Part model, mm, in its own coordinate system. A direction names the side the tool comes from. Round coordinates to 2 decimals unless told otherwise and drop trailing zeros. Loops run counter-clockwise (first coordinate to the right, second up) from the corner with the lowest first, then second, coordinate; pieces in that order, holes last. Notation, with made-up numbers: M 52,76.5 L 100,76.5 A36 cw 100,112.5 Z; hole C 83,12 d10. An arc over 180 degrees is marked long. Put each result on its own line as item: value. Start each with the question number.
1) Slice it at A-A on y = -114.5. Give the cut face in (x, z).
2) Which spindle directions (+Z, -Z, +X, -X, +Y, -Y) get a long thin tool onto all of the face, cutting with end or side? Do faces 4 (the flat face through (-44.999, -174, 21)), 5 (the flat face through (-84.999, -174, 20)), 6 (the cylindrical face through (-133.47, -115.27, 21.75)), 7 (the flat face through (-85.999, 4, 21)), 8 (the flat face through (-10, -130.481, 3)). Say none if no direction does.
3) Pull direction Y, two halves, no side cores. Call faces 1 (the flat face through (-75, -104, 15)), 2 (the cylindrical face through (-110.353, -64.656, 3.372)), 3 (the cylindrical face through (-142.69, -115.27, 1.6)): +Y half, -Y half, draft (parallel to the pull), parting line (faces both ways), or undercut.
4) Slice it at D-D on y = -136.5. Give the cut face in (x, z), then the cut area to 3 significant figures.
5) Slice it at C-C on x = -158. Give the cut face in (y, z).
6) Probe line 1 along Y through (x, z) = (-78, 43.5); line 2 along Z through (x, y) = (-26, -109); line 3 along X through (y, z) = (-83.5, 37). List the from-to ranges inside material, lowest first.
7) Slice it at B-B on y = -67.5. Give the cut face in (x, z).
8) Drop flat-ended pins along their axis: pin 1 Ø5.5 at (y, z) = (-101, 5) entering from -X; pin 2 Ø3.5 at (x, z) = (-9.5, 4.5) entering from -Y; pin 3 Ø12 at (y, z) = (-172, 25) entering from +X. Give the stop position or say it passes through.
```python
from build123d import *

# Parameters (mm, degrees)
EXTRUDE_1_DEPTH     = 6.84
EXTRUDE_2_DEPTH     = 12
SKETCH_3_R          = 26.5
EXTRUDE_3_DEPTH     = 48.5
SKETCH_4_R          = 31.5
EXTRUDE_4_DEPTH     = 5.63
SKETCH_5_R          = 21
CUT_EXTRUDE_1_DEPTH = 9.13
SKETCH_6_R          = 21
CUT_EXTRUDE_2_DEPTH = 2.92
SKETCH_7_R          = 16
SKETCH_9_R          = 21
SKETCH_8_R          = 16
SKETCH_10_R         = 17
CUT_EXTRUDE_3_DEPTH = 13.29
SKETCH_11_R         = 6
CUT_EXTRUDE_4_DEPTH = 42.92
EXTRUDE_5_DEPTH     = 15
SKETCH_13_R         = 5.5
CUT_EXTRUDE_5_DEPTH = 15
EXTRUDE_6_DEPTH     = 15
SKETCH_16_R         = 5.5
CUT_EXTRUDE_6_DEPTH = 15


with BuildPart() as part:
    # 스케치1 → 보스-돌출1 (new body)
    with BuildSketch(Plane.XY):
        with BuildLine():
            Line((-34.998826986, -181.181097978), (-34.998826986, -140.481097978))
            ThreePointArc((-34.998826986, -140.481097978), (-32.069894798, -133.410030166), (-24.998826986, -130.481097978))
            Line((-24.998826986, -130.481097978), (5.001173014, -130.481097978))
            Line((5.001173014, -130.481097978), (5.001173014, -47.181097978))
            Line((5.001173014, -47.181097978), (-25.998826986, -47.181097978))
            ThreePointArc((-25.998826986, -47.181097978), (-33.069894798, -44.25216579), (-35.998826986, -37.181097978))
            Line((-35.998826986, -37.181097978), (-35.998826986, 11.818902022))
            Line((-35.998826986, 11.818902022), (-95.998826986, 11.818902022))
            Line((-95.998826986, 11.818902022), (-95.998826986, -48.181097978))
            ThreePointArc((-95.998826986, -48.181097978), (-110.502915378, -64.929776001), (-116.68226469, -86.206581157))
            Line((-116.68226469, -86.206581157), (-116.68226469, -87.311097978))
            Line((-116.68226469, -87.311097978), (-134.998826986, -87.311097978))
            Line((-134.998826986, -87.311097978), (-134.998826986, -121.181097978))
            Line((-134.998826986, -121.181097978), (-104.998826986, -121.181097978))
            ThreePointArc((-104.998826986, -121.181097978), (-97.927759174, -124.110030166), (-94.998826986, -131.181097978))
            Line((-94.998826986, -131.181097978), (-94.998826986, -181.181097978))
            Line((-94.998826986, -181.181097978), (-34.998826986, -181.181097978))
        make_face()
    extrude(amount=EXTRUDE_1_DEPTH)

    # 스케치2 → 보스-돌출2 (add)
    with BuildSketch(Plane.XZ.offset(121.181097978)):
        with BuildLine():
            Line((-114.998826986, 0), (-114.998826986, 15.74))
            ThreePointArc((-114.998826986, 15.74), (-116.46329308, 19.275533906), (-119.998826986, 20.74))
            Line((-119.998826986, 20.74), (-129.093412943, 20.74))
            ThreePointArc((-129.093412943, 20.74), (-133.528440233, 21.777269783), (-137.043403564, 24.673893413))
            Line((-137.043403564, 24.673893413), (-164.048836366, 60.066106587))
            ThreePointArc((-164.048836366, 60.066106587), (-178.064933574, 61.949990621), (-179.948817607, 47.933893413))
            Line((-179.948817607, 47.933893413), (-147.876203482, 5.900840119))
            ThreePointArc((-147.876203482, 5.900840119), (-142.603758486, 1.555904675), (-135.951217551, 0))
            Line((-135.951217551, 0), (-114.998826986, 0))
        make_face()
    extrude(amount=-EXTRUDE_2_DEPTH)

    # 스케치3 → 보스-돌출3 (add)
    with BuildSketch(Plane.XY.offset(6.84)):
        with Locations(Location((-64.998826986, -91.181097978, 0), (0, 0, 180))):
            Circle(SKETCH_3_R)
    extrude(amount=EXTRUDE_3_DEPTH)

    # 스케치4 → 보스-돌출4 (add)
    with BuildSketch(Plane.XY.offset(6.84)):
        with Locations((-64.998826986, -91.181097978)):
            Circle(SKETCH_4_R)
    extrude(amount=EXTRUDE_4_DEPTH)

    # 스케치5 → 컷-돌출1 (cut)
    with BuildSketch(Plane.XY.offset(55.34)):
        with Locations((-64.998826986, -91.181097978)):
            Circle(SKETCH_5_R)
    extrude(amount=-CUT_EXTRUDE_1_DEPTH, mode=Mode.SUBTRACT)

    # 스케치6 → 컷-돌출2 (cut)
    with BuildSketch(Plane.XY.offset(46.21)):
        with Locations((-64.998826986, -91.181097978)):
            Circle(SKETCH_6_R)
    extrude(amount=-CUT_EXTRUDE_2_DEPTH, mode=Mode.SUBTRACT)

    # 스케치7 → section 0 of loft_1
    with BuildSketch(Plane.XY.offset(28.29), mode=Mode.PRIVATE) as loft_1_s0:
        with Locations((-64.998826986, -91.181097978)):
            Circle(SKETCH_7_R)
    # loft up to a face of the part (loft_1)
    loft([loft_1_s0.sketch, Face(Wire([part.edges().sort_by_distance((-79.374316211, -75.872756802, 43.29))[0]]))], mode=Mode.SUBTRACT)

    # 스케치9 → 컷-로프트3 section 0
    with BuildSketch(Plane(origin=(0, 0, 0), x_dir=(-1, 0, 0), z_dir=(0, 0, -1))):
        with Locations((64.998826986, -91.181097978)):
            Circle(SKETCH_9_R)
    # 스케치8 → 컷-로프트3 section 1
    with BuildSketch(Plane(origin=(0, 0, 15), x_dir=(-1, 0, 0), z_dir=(0, 0, -1))):
        with Locations((64.998826986, -91.181097978)):
            Circle(SKETCH_8_R)
    loft(mode=Mode.SUBTRACT)

    # 스케치10 → 컷-돌출3 (cut)
    with BuildSketch(Plane(origin=(0, 0, 15), x_dir=(-1, 0, 0), z_dir=(0, 0, -1))):
        with Locations((64.998826986, -91.181097978)):
            Circle(SKETCH_10_R)
    extrude(amount=-CUT_EXTRUDE_3_DEPTH, mode=Mode.SUBTRACT)

    # 스케치11 → 컷-돌출4 (cut)
    with BuildSketch(Plane(origin=(0, -109.181097978, 0), x_dir=(1, 0, 0), z_dir=(0, 1, 0))):
        with Locations(Location((-171.998826986, -54, 0), (0, 0, 180))):
            Circle(SKETCH_11_R)
    extrude(amount=-CUT_EXTRUDE_4_DEPTH, mode=Mode.SUBTRACT)

    # 스케치12 → 보스-돌출5 (add)
    with BuildSketch(Plane.XZ.offset(181.181097978)):
        with BuildLine():
            Line((-84.998826986, 6.84), (-84.998826986, 34.091376239))
            ThreePointArc((-84.998826986, 34.091376239), (-64.998826986, 54.091376239), (-44.998826986, 34.091376239))
            Line((-44.998826986, 34.091376239), (-44.998826986, 6.84))
            Line((-44.998826986, 6.84), (-84.998826986, 6.84))
        make_face()
    extrude(amount=-EXTRUDE_5_DEPTH)

    # 스케치13 → 컷-돌출5 (cut)
    with BuildSketch(Plane.XZ.offset(181.181097978)):
        with Locations(Location((-64.998826986, 34.091376239, 0), (0, 0, 270))):
            Circle(SKETCH_13_R)
    extrude(amount=-CUT_EXTRUDE_5_DEPTH, mode=Mode.SUBTRACT)

    # 스케치15 → 보스-돌출6 (add)
    with BuildSketch(Plane(origin=(0, 11.818902022, 0), x_dir=(1, 0, 0), z_dir=(0, 1, 0))):
        with BuildLine():
            Line((-85.998826986, -6.84), (-85.998826986, -35.286448376))
            ThreePointArc((-85.998826986, -35.286448376), (-65.998826986, -55.286448376), (-45.998826986, -35.286448376))
            Line((-45.998826986, -35.286448376), (-45.998826986, -6.84))
            Line((-45.998826986, -6.84), (-85.998826986, -6.84))
        make_face()
    extrude(amount=-EXTRUDE_6_DEPTH)

    # 스케치16 → 컷-돌출6 (cut)
    with BuildSketch(Plane(origin=(0, 11.818902022, 0), x_dir=(1, 0, 0), z_dir=(0, 1, 0))):
        with Locations(Location((-65.998826986, -35.286448376, 0), (0, 0, 270))):
            Circle(SKETCH_16_R)
    extrude(amount=-CUT_EXTRUDE_6_DEPTH, mode=Mode.SUBTRACT)


solid = part.part
```
Recorded:
1. outline: M -179.95,47.93 L -147.88,5.9 A15 ccw -135.95,0 L 5,0 L 5,6.84 L -43.82,6.84 L -43.82,12.47 L -52.41,12.47 L -52.41,55.34 L -77.59,55.34 L -77.59,12.47 L -86.18,12.47 L -86.18,6.84 L -115,6.84 L -115,15.74 A5 ccw -120,20.74 L -129.09,20.74 A10 cw -137.04,24.67 L -164.05,60.07 A10 ccw Z; hole C -172,54 d12
2. face 4: +Z, +X, -Y
2. face 5: +Z, -X, -Y
2. face 6: +Z, +Y, -Y
2. face 7: +Z, -X, +Y
2. face 8: +Z, -Z, +X, -Y
3. face 1: undercut
3. face 2: +Y half
3. face 3: draft
4. outline: M -95,0 L -34.17,0 L -34.17,6.84 L -95,6.84 Z
4. area: 416 mm2
5. outline: M -121.18,19.17 L -109.18,19.17 L -109.18,52.14 L -121.18,52.14 Z
6. line 1: y = -181.18 to -166.18, -114.27 to -107.67, -74.69 to -68.09, -3.18 to 11.82
6. line 2: z = 0 to 6.84
6. line 3: x = -90.36 to -82.27, -47.73 to -39.64
7. outline: M -111.81,0 L 5,0 L 5,6.84 L -44.23,6.84 L -44.23,12.47 L -53.11,12.47 L -53.11,55.34 L -76.89,55.34 L -76.89,12.47 L -85.77,12.47 L -85.77,6.84 L -111.81,6.84 Z
8. pin 1: stops at x = -135
8. pin 2: stops at y = -130.48
8. pin 3: stops at x = -45
